Answer from the drawing. Dimensions are ordinates in mm from the lowest x, y and z of the part. Coordinates: 2 decimals unless noted, no trailing zeros. Write each loop counter-clockwise with the first axis right and the second up, starting at its lowest first coordinate (ties: lowest second). Pieces come first, ordered by that corner, then holes.
(1) Find the intervals of material crossed by probe 1 along X at (y, z) = (2, 14); probe 2 along Z at (x, y) = (7, 4.25); probe 3 along Z at (x, y) = (4, 2.5), in increasing order.
(2) Given pin 1 (2.5 mm diameter, centred on x = 45, z = 5, fed in from -Y); pin 2 (4 mm diameter, centred on x = 4.5, z = 5.5, fed in from +Y) (3 decimals), each flat-ended and moving along its own axis, determine where each tip first touches the part or whether it passes through.
(3) Section B-B on y = 1.75 is taken. State how many separate pieces and enclosed holes the cut face has, then the cut area to 3 significant figures.
(4) Section A-A on x = 15.5 is taken. Write down the section's boundary in (y, z).
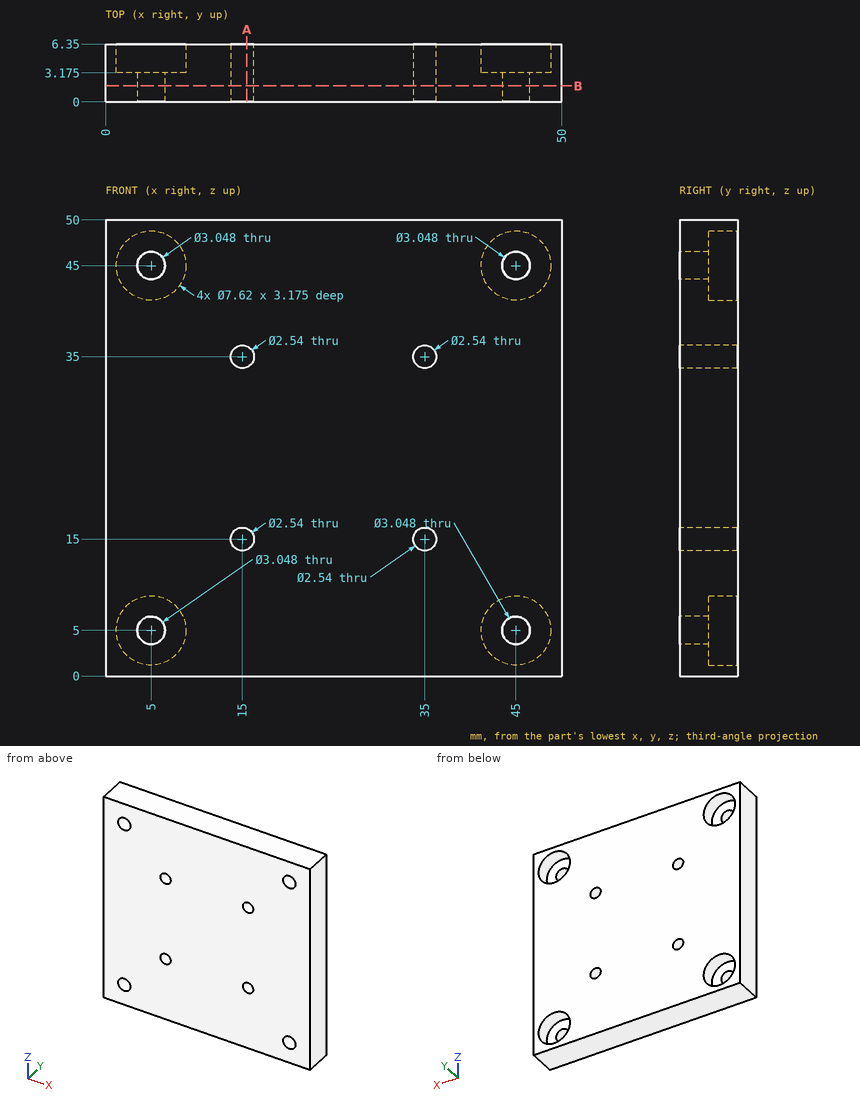
Response:
1. probe 1: x = 0 to 14.22, 15.78 to 34.22, 35.78 to 50
1. probe 2: z = 0 to 1.76, 8.24 to 41.76, 48.24 to 50
1. probe 3: z = 0 to 3.85, 6.15 to 43.85, 46.15 to 50
2. pin 1: passes through
2. pin 2: stops at y = 3.175
3. separate pieces: 1
3. enclosed holes: 8
3. area: 2,450 mm2
4. outline: (0, 0) - (6.35, 0) - (6.35, 13.83) - (0, 13.83) - close; (0, 16.17) - (6.35, 16.17) - (6.35, 33.83) - (0, 33.83) - close; (0, 36.17) - (6.35, 36.17) - (6.35, 50) - (0, 50) - close
